Could you check a few things on this model? Use its own coordinates, in mm. Give positions to 0.01 mm unless a question says otherwise; leave off trailing zeros. Order: outer loops, then holes, each group sorted by start corner. A loop starts at its lowest first (then second) coordinate and runs counter-clockwise, first axis right, second up. Notation, with made-up numbers: M 73.25,65.5 L 122.25,65.5 A26 ccw 122.25,103.5 Z; hole C -25.5,-4.5 d8. An arc over 180 degrees is marked long. Use a Markdown table: item, result. Add a question column.
Item 1: Suppose I cut it at C-C on x = -65. Write out the boundary of the cut face in (y, z).
Item 2: If we mould it in two halves opening along Y, with no side actions, what happens to faces 1 (the face through (-1, -85, 0)), 2 (the face through (63.441, -37.997, -0.089)), 3 (the face through (75, -1, 0)), 4 (the face through (-44.27, 71.7, -0.09))? For each: released by +Y, released by -Y, zero draft, split by the parting line, or undercut.
Item 3: I'm going to push a flat-ended pin straight in: pin 1 Ø4 at (x, y) = (-65, 35) entering from +Z. Where does the tip first touch, or does it pass through?
Item 4: Suppose I cut it at A-A on y = 75. Write out the boundary of the cut face in (x, z).
Item 5: If I drill on L1, parallel to Y at x = 45, z = 0.5; L2, parallel to X at y = 76.5, z = 4.25; L3, parallel to X at y = -73, z = 3.5, over which ranges is the centre line in solid material (lowest first)? Write a range as from..to.
Item 6: Suppose I cut it at B-B on z = -2.25. Count the separate pieces of the cut face and the enclosed holes in it, plus the area to 3 significant figures.
from build123d import *

# Parameters (mm, degrees)
CROQUIS1_W                    = 150
CROQUIS1_H                    = 170
SALIENTE_EXTRUIR1_DEPTH       = 6.35
TALADRO_DE_MARGEN_PARA_1_41_D = 6.7564


with BuildPart() as part:
    # Croquis1 → Saliente-Extruir1 (new, symmetric)
    with BuildSketch(Plane.XY):
        Rectangle(CROQUIS1_W, CROQUIS1_H)
    extrude(amount=SALIENTE_EXTRUIR1_DEPTH, both=True)

    # Taladro de margen para 1/41 (through all)
    with Locations(Plane.XY.offset(6.35)):
        with Locations((65, 75), (65, 35), (45, 35), (45, 75), (45, -75), (45, -35), (65, -35), (65, -75), (-65, -75), (-65, -35), (-45, -35), (-45, -75), (-45, 75), (-45, 35), (-65, 35), (-65, 75)):
            Hole(TALADRO_DE_MARGEN_PARA_1_41_D / 2)


solid = part.part
Findings below:
| question | item | result |
|---|---|---|
| 1 | outline | M -85,-6.35 L -78.38,-6.35 L -78.38,6.35 L -85,6.35 Z; M -71.62,-6.35 L -38.38,-6.35 L -38.38,6.35 L -71.62,6.35 Z; M -31.62,-6.35 L 31.62,-6.35 L 31.62,6.35 L -31.62,6.35 Z; M 38.38,-6.35 L 71.62,-6.35 L 71.62,6.35 L 38.38,6.35 Z; M 78.38,-6.35 L 85,-6.35 L 85,6.35 L 78.38,6.35 Z |
| 2 | face 1 | released by -Y |
| 2 | face 2 | undercut |
| 2 | face 3 | zero draft |
| 2 | face 4 | undercut |
| 3 | pin 1 | passes through |
| 4 | outline | M -75,-6.35 L -68.38,-6.35 L -68.38,6.35 L -75,6.35 Z; M -61.62,-6.35 L -48.38,-6.35 L -48.38,6.35 L -61.62,6.35 Z; M -41.62,-6.35 L 41.62,-6.35 L 41.62,6.35 L -41.62,6.35 Z; M 48.38,-6.35 L 61.62,-6.35 L 61.62,6.35 L 48.38,6.35 Z; M 68.38,-6.35 L 75,-6.35 L 75,6.35 L 68.38,6.35 Z |
| 5 | L1 | y = -85..-78.38, -71.62..-38.38, -31.62..31.62, 38.38..71.62, 78.38..85 |
| 5 | L2 | x = -75..-68.03, -61.97..-48.03, -41.97..41.97, 48.03..61.97, 68.03..75 |
| 5 | L3 | x = -75..-67.72, -62.28..-47.72, -42.28..42.28, 47.72..62.28, 67.72..75 |
| 6 | separate pieces | 1 |
| 6 | enclosed holes | 16 |
| 6 | area | 24,900 mm^2 |
